```python
from build123d import *

# Parameters (mm, degrees)
ESBO_O1_R                = 31.5
ESBO_O1_R_2              = 30.5
RESSALTO_EXTRUS_O1_DEPTH = 50
ESBO_O2_R                = 32.5
ESBO_O2_R_2              = 30.5
RESSALTO_EXTRUS_O2_DEPTH = 20
ESBO_O3_R                = 31.5
ESBO_O3_R_2              = 30.5
RESSALTO_EXTRUS_O3_DEPTH = 50
RESSALTO_EXTRUS_O4_START = -5
ESBO_O6_R                = 30.5
RESSALTO_EXTRUS_O4_DEPTH = 5


with BuildPart() as part:
    # Esbo_o1 → Ressalto-extrus_o1 (new body)
    with BuildSketch(Plane(origin=(0, 0, 0), x_dir=(1, 0, 0), z_dir=(0, 1, 0))):
        with Locations(Location((0, 0, 0), (0, 0, 270))):
            Circle(ESBO_O1_R)
        with Locations(Location((0, 0, 0), (0, 0, 270))):
            Circle(ESBO_O1_R_2, mode=Mode.SUBTRACT)
    extrude(amount=RESSALTO_EXTRUS_O1_DEPTH)


with BuildPart() as body_2:
    # Esbo_o2 → Ressalto-extrus_o2 (new body)
    with BuildSketch(Plane(origin=(0, 50, 0), x_dir=(1, 0, 0), z_dir=(0, 1, 0))):
        with Locations(Location((0, 0, 0), (0, 0, 270))):
            Circle(ESBO_O2_R)
        with Locations(Location((0, 0, 0), (0, 0, 270))):
            Circle(ESBO_O2_R_2, mode=Mode.SUBTRACT)
    extrude(amount=RESSALTO_EXTRUS_O2_DEPTH)



with BuildPart() as body_3:
    # Esbo_o3 → Ressalto-extrus_o3 (new body)
    with BuildSketch(Plane(origin=(0, 70, 0), x_dir=(1, 0, 0), z_dir=(0, 1, 0))):
        with Locations(Location((0, 0, 0), (0, 0, 270))):
            Circle(ESBO_O3_R)
        with Locations(Location((0, 0, 0), (0, 0, 270))):
            Circle(ESBO_O3_R_2, mode=Mode.SUBTRACT)
    extrude(amount=RESSALTO_EXTRUS_O3_DEPTH)


with BuildPart() as body_2_1:
    add(body_2.part)

    add(body_3.part)  # Ressalto-extrus_o4 merges body 3
    # Esbo_o6 → Ressalto-extrus_o4 (add)
    with BuildSketch(Plane(origin=(0, 70, 0), x_dir=(1, 0, 0), z_dir=(0, 1, 0)).offset(RESSALTO_EXTRUS_O4_START)):
        with Locations(Location((0, 0, 0), (0, 0, 270))):
            Circle(ESBO_O6_R)
    extrude(amount=RESSALTO_EXTRUS_O4_DEPTH)


with BuildPart() as part_1:
    add(part.part)

    # Combinar3: union body 2
    add(body_2_1.part)


solid = part_1.part
```
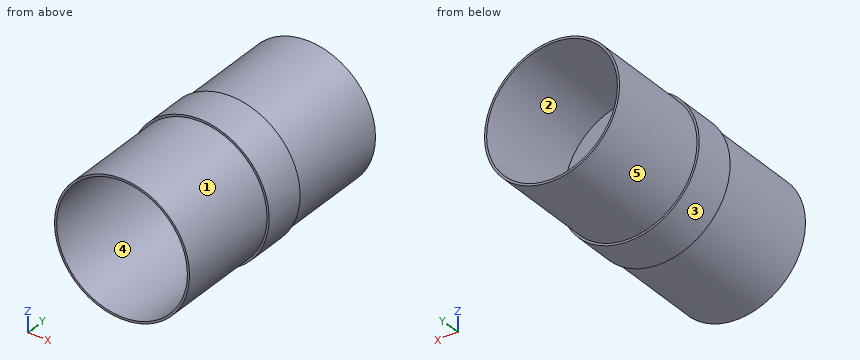
Input: part model. Units: mm. Frame: model coordinates. Face numbers are marked on the shaded views. A direction names the side the tool comes from. Give positions to 0.01 mm unless a question says otherwise; leave off trailing zeros. Loops run counter-clockwise (first coordinate to the right, second up) from the corner with the lowest first, then second, coordinate; pieces in that order, holes last.
1) Section query B-B on y = 55.5. Return the cut outline in (x, z).
A:
outline: circle Ø65 at (0, 0); hole circle Ø61 at (0, 0)
2) Contact query for flat-ended pins moving along their axis: pin 1 (6 mm diameter, centred on x = -10, y = 105.5, fed in from +Z); pin 2 (6 mm diameter, centred on y = 27.5, z = 12, fed in from +X); pin 3 (4 mm diameter, centred on x = 16, y = 82, fed in from +Z). Output: stop coordinate, or through.
A:
pin 1: stops at z = 30.71
pin 2: stops at x = 30.19
pin 3: stops at z = 28.22
3) Mould query, pull axis Z, two halves, no side actions, for the marked faces 4 and 5. Classes: released by +Z, released by -Z, zero draft, split by the parting line, or undercut.
A:
face 4: undercut
face 5: split by the parting line
4) Reachability of the marked faces 1, 2 and 3 from +Z, -Z, +X, -X, +Y, -Y: full face, straight path, thin tool, end or side. Return the list, or none.
A:
face 1: -Y
face 2: +Y
face 3: +Y, -Y
5) Line query: L1, parallel to X at y = 24, z = 0; L2, parallel to Y at x = -10.5, z = 3.5; L3, parallel to X at y = 64, z = 27. Output: solid intervals per line, ascending.
A:
L1: x = -31.5 to -30.5, 30.5 to 31.5
L2: y = 65 to 70
L3: x = -18.09 to -14.19, 14.19 to 18.09
6) Section query C-C on z = 0. Return the cut outline in (x, y), and give its area (3 significant figures).
A:
outline: (-32.5, 50) - (-31.5, 50) - (-31.5, 0) - (-30.5, 0) - (-30.5, 65) - (30.5, 65) - (30.5, 0) - (31.5, 0) - (31.5, 50) - (32.5, 50) - (32.5, 70) - (31.5, 70) - (31.5, 120) - (30.5, 120) - (30.5, 70) - (-30.5, 70) - (-30.5, 120) - (-31.5, 120) - (-31.5, 70) - (-32.5, 70) - close
area: 585 mm2
7) Section query A-A on x = 0. Return the cut outline in (y, z).
A:
outline: (0, -31.5) - (50, -31.5) - (50, -32.5) - (70, -32.5) - (70, -31.5) - (120, -31.5) - (120, -30.5) - (70, -30.5) - (70, 30.5) - (120, 30.5) - (120, 31.5) - (70, 31.5) - (70, 32.5) - (50, 32.5) - (50, 31.5) - (0, 31.5) - (0, 30.5) - (65, 30.5) - (65, -30.5) - (0, -30.5) - close
8) Section query D-D on y = 30.5. Return the cut outline in (x, z), and give its area (3 significant figures).
A:
outline: circle Ø63 at (0, 0); hole circle Ø61 at (0, 0)
area: 195 mm2
